from build123d import *

# Parameters (mm, degrees)
F0_W     = 50.8
F0_H     = 50.8
F1_DEPTH = 50.8
F2_W     = 38.1
F2_H     = 25.4
F3_DEPTH = 25.4


with BuildPart() as f1:
    # F0 (on Top) → F1 (new body)
    with BuildSketch(Plane.XY):
        with Locations((3.653681, -0.464274)):
            Rectangle(F0_W, F0_H)
    extrude(amount=F1_DEPTH)

    # F2 (on face) → F3 (cut)
    with BuildSketch(Plane.XZ.offset(25.864274)):
        with Locations((10.003681, 12.7)):
            Rectangle(F2_W, F2_H)
    extrude(amount=-F3_DEPTH, mode=Mode.SUBTRACT)


solid = f1.part
Verification items for the finished model (mm, model axes). A direction names the side the tool comes from. Coordinates: 2 decimals unless noted, no trailing zeros. Order: outer loops, then holes, each group sorted by start corner. A loop starts at its lowest first (then second) coordinate and runs counter-clockwise, first axis right, second up.
1. Scan lines: line 1 (Z direction, x = 5, y = -6.5); line 2 (Y direction, x = 13.5, z = 14.5); line 3 (X direction, y = -22.5, z = 2.5). Record each from-to range of solid material in increasing order.
Results found:
line 1: z = 25.4 to 50.8
line 2: y = -0.46 to 24.94
line 3: x = -21.75 to -9.05
2. Set-up check for faces 1 (the face through (10, -13, 25.4)), 2 (the face through (-2, 6, 0)): record each of +Z, -Z, +X, -X, +Y, -Y from which the full face is reachable in a straight line by a thin tool's end or side.
Results found:
face 1: -Z, +X, -Y
face 2: -Z, +X, -X, +Y, -Y
3. Sectioned sample at A-A, the plane y = -23. Record the cut outline in (x, z), and give its area (3 significant figures).
Results found:
outline: (-21.75, 0) - (-9.05, 0) - (-9.05, 25.4) - (29.05, 25.4) - (29.05, 50.8) - (-21.75, 50.8) - close
area: 1,610 mm2
4. Sectioned sample at B-B, the plane z = 21.5. Record the cut outline in (x, y), and give its area (3 significant figures).
Results found:
outline: (-21.75, -25.86) - (-9.05, -25.86) - (-9.05, -0.46) - (29.05, -0.46) - (29.05, 24.94) - (-21.75, 24.94) - close
area: 1,610 mm2
5. Go/stop test with flat-tipped pins: pin 1 Ø20.5 at (y, z) = (-11.5, 8.5) entering from +X; pin 2 Ø12.5 at (x, y) = (11.5, -16.5) entering from -Z; pin 3 Ø20.5 at (x, z) = (12.5, 9) entering from -Y; pin 4 Ø1 at (x, y) = (-2, 4.5) entering from -Z. Record where each tip stops, or that it passes through.
Results found:
pin 1: stops at x = -9.05
pin 2: stops at z = 25.4
pin 3: stops at y = -0.46
pin 4: stops at z = 0
